```python
from build123d import *

# Parameters (mm, degrees)
F0_W     = 175
F0_H     = 12.7
F1_DEPTH = 12.7
F2_W     = 38.1
F2_H     = 12.7
F3_DEPTH = 6.35
F4_W     = 168
F4_H     = 2.5
F5_DEPTH = 10.16


with BuildPart() as f1:
    # F0 (on Top) → F1 (new body)
    with BuildSketch(Plane.XY):
        Rectangle(F0_W, F0_H)
    extrude(amount=F1_DEPTH)

    # F2 (on face) → F3 (join)
    with BuildSketch(Plane(origin=(0, 0, 0), x_dir=(1, 0, 0), z_dir=(0, 0, -1))):
        with Locations((0, -12.7)):
            Rectangle(F2_W, F2_H)
        with Locations((0, 12.7)):
            Rectangle(F2_W, F2_H)
    extrude(amount=-F3_DEPTH)

    # F4 (on face) → F5 (cut)
    with BuildSketch(Plane.XY.offset(12.7)):
        Rectangle(F4_W, F4_H)
    extrude(amount=-F5_DEPTH, mode=Mode.SUBTRACT)


solid = f1.part
```
Model file for the job. Use its own axes, mm. A direction names the side the tool comes from. Give positions to 0.01 mm unless a question says otherwise; leave off trailing zeros. Loops run counter-clockwise (first coordinate to the right, second up) from the corner with the lowest first, then second, coordinate; pieces in that order, holes last. Notation, with made-up numbers: (-26.75, 43) -> (-14.75, 43) arc R18 ccw to (-14.75, 65) -> close; hole circle Ø8 at (22, -12). An arc over 180 degrees is marked (long way). Use CSV: the item, a comma, the result in double quotes. Start each with the question number.
1) Slice it at C-C on x = -6. Give the cut face in (y, z), plus the area to 3 significant figures.
2) Flat gauge pins, fed straight in: pin 1 Ø1.9 at (y, z) = (-15.5, 4.5) entering from +X; pin 2 Ø1 at (x, z) = (-24, 11) entering from -Y; pin 3 Ø4 at (x, z) = (-20, 7.5) entering from -Y; pin 4 Ø3 at (y, z) = (15, 3) entering from -X. Where does each tip first touch, or does it go through?
3) Wall check: line 1 (Y direction, x = -71.5, z = 4.25); line 2 (X direction, y = 11, z = 4); line 3 (Y direction, x = -10.5, z = 5). Give the ranges that are in metal, low to high.
4) Tool access for faces 4 (the flat face through (-19.05, -13, 3)), 5 (the flat face through (0, -13, 6.35)), 6 (the flat face through (19.05, -13, 3)): list every direction of +Z, -Z, +X, -X, +Y, -Y with a clear straight run to the whole face (end or side of a thin tool).
5) Mould opens along Y. For faces 1 (the flat face through (0, 19.05, 3)), 2 (the flat face through (-1, -1.25, 8)), 3 (the flat face through (87.5, 0, 6)) say: released by +Y, released by -Y, zero draft, split by the parting line, or undercut.
6) Slice it at B-B on x = -34.5. Give the cut face in (y, z), plus the area to 3 significant figures.
7) Slice it at A-A on z = 9.25. Give the cut face in (x, y).
Computed values:
1,outline,"(-19.05, 0) -> (19.05, 0) -> (19.05, 6.35) -> (6.35, 6.35) -> (6.35, 12.7) -> (1.25, 12.7) -> (1.25, 2.54) -> (-1.25, 2.54) -> (-1.25, 12.7) -> (-6.35, 12.7) -> (-6.35, 6.35) -> (-19.05, 6.35) -> close"
1,area,"297 mm^2"
2,pin 1,"stops at x = 19.05"
2,pin 2,"stops at y = -6.35"
2,pin 3,"stops at y = -19.05"
2,pin 4,"stops at x = -19.05"
3,line 1,"y = -6.35 to -1.25, 1.25 to 6.35"
3,line 2,"x = -19.05 to 19.05"
3,line 3,"y = -19.05 to -1.25, 1.25 to 19.05"
4,face 4,"+Z, -Z, -X, -Y"
4,face 5,"+Z, +X, -X, -Y"
4,face 6,"+Z, -Z, +X, -Y"
5,face 1,"released by +Y"
5,face 2,"undercut"
5,face 3,"zero draft"
6,outline,"(-6.35, 0) -> (6.35, 0) -> (6.35, 12.7) -> (1.25, 12.7) -> (1.25, 2.54) -> (-1.25, 2.54) -> (-1.25, 12.7) -> (-6.35, 12.7) -> close"
6,area,"136 mm^2"
7,outline,"(-87.5, -6.35) -> (87.5, -6.35) -> (87.5, 6.35) -> (-87.5, 6.35) -> close; hole (-84, -1.25) -> (84, -1.25) -> (84, 1.25) -> (-84, 1.25) -> close"
